Source: three-view drawing plus pictorial views. Frame: mm from the lowest corner of the part. Round coordinates to 2 decimals unless told otherwise and drop trailing zeros. Loops run counter-clockwise (first coordinate to the right, second up) from the corner with the lowest first, then second, coordinate; pieces in that order, holes last. Notation, with made-up numbers: M 12,-19 L 70,-19 A21 ccw 70,19 Z; hole C -39.75,-20 d8. An arc over 180 degrees is marked long. Answer as a JSON object with one key per item and string values.
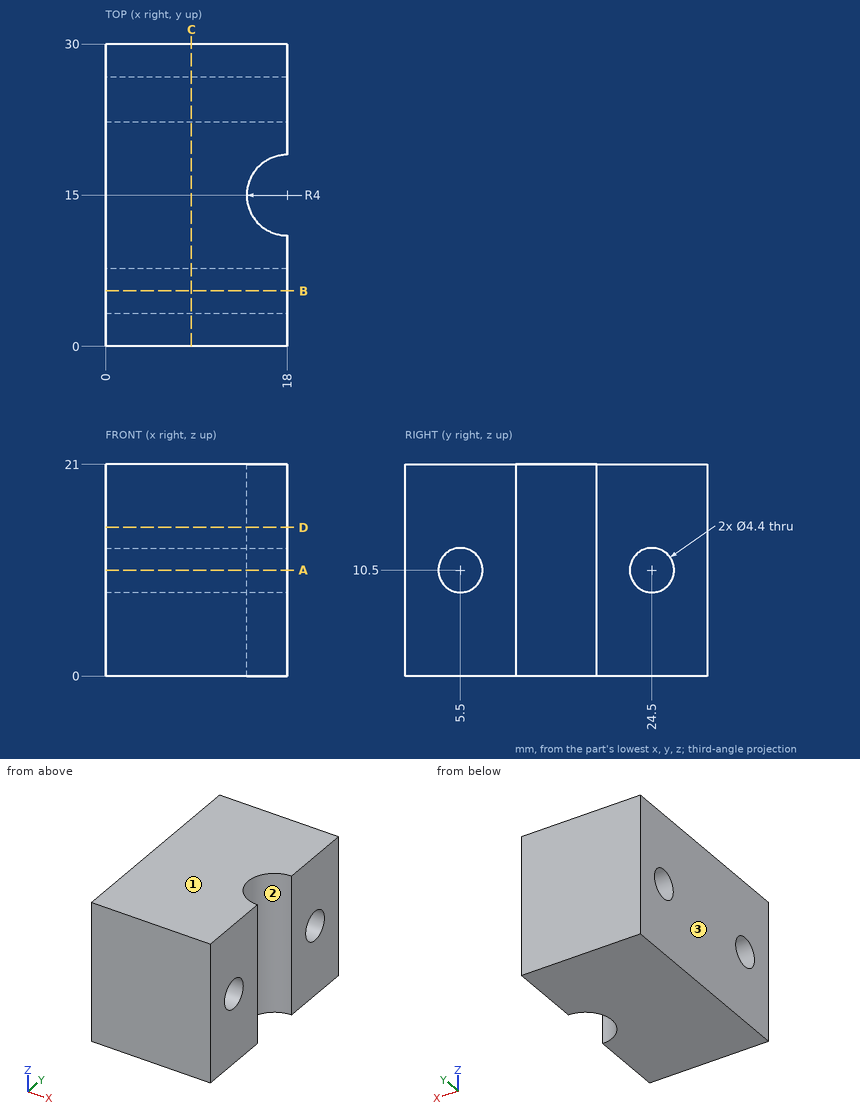
1) Line query: probe 1 along Z at (x, y) = (5.25, 5.5); probe 2 along Y at (x, z) = (6.75, 11.75); probe 3 along Z at (x, y) = (4, 22.5). Output: solid intervals per line, ascending.
Geometry results:
{"probe 1": "0 to 8.3, 12.7 to 21", "probe 2": "0 to 3.69, 7.31 to 22.69, 26.31 to 30", "probe 3": "0 to 9.58, 11.42 to 21"}
2) Pull-direction query (X, two-part tool) for the marked faces 1, 2 and 3; classes: +X half, -X half, draft (parallel to the pull), parting line (faces both ways), or undercut.
Geometry results:
{"face 1": "draft", "face 2": "+X half", "face 3": "-X half"}
3) First-contact query: pin 1 (4 mm diameter, centred on y = 5.5, z = 10.5, fed in from +X). Flat tip, straight axial feed; report the tip coordinate or a pass-through.
Geometry results:
{"pin 1": "through"}
4) Cut plane D-D on z = 14.75. Return the cut outline in (x, y), and give its area (3 significant figures).
Geometry results:
{"outline": "M 0,0 L 18,0 L 18,11 A4 cw 18,19 L 18,30 L 0,30 Z", "area": "515 mm2"}
5) Cut plane A-A on z = 10.5. Return the cut outline in (x, y), and give its area (3 significant figures).
Geometry results:
{"outline": "M 0,0 L 18,0 L 18,3.3 L 0,3.3 Z; M 0,7.7 L 18,7.7 L 18,11 A4 cw 18,19 L 18,22.3 L 0,22.3 Z; M 0,26.7 L 18,26.7 L 18,30 L 0,30 Z", "area": "356 mm2"}
6) Cut plane B-B on y = 5.5. Return the cut outline in (x, z), and give its area (3 significant figures).
Geometry results:
{"outline": "M 0,0 L 18,0 L 18,8.3 L 0,8.3 Z; M 0,12.7 L 18,12.7 L 18,21 L 0,21 Z", "area": "299 mm2"}
7) Cut plane C-C on x = 8.5. Return the cut outline in (y, z), and give its area (3 significant figures).
Geometry results:
{"outline": "M 0,0 L 30,0 L 30,21 L 0,21 Z; hole C 5.5,10.5 d4.4; hole C 24.5,10.5 d4.4", "area": "600 mm2"}
